Build history of the part. All positions in model axes, mm. Face numbers are marked on the shaded views. A direction names the side the tool comes from. Round coordinates to 2 decimals unless told otherwise and drop trailing zeros. Loops run counter-clockwise (first coordinate to the right, second up) from the corner with the lowest first, then second, coordinate; pieces in that order, holes last. Notation, with made-up numbers: (-35, 4.5) - (13, 4.5) arc R7 ccw to (13, 9.5) - close; hole circle Ø6 at (59, -21.75). An arc over 180 degrees is marked (long way). Put each result on its own line as item: value. Start each with the question number.
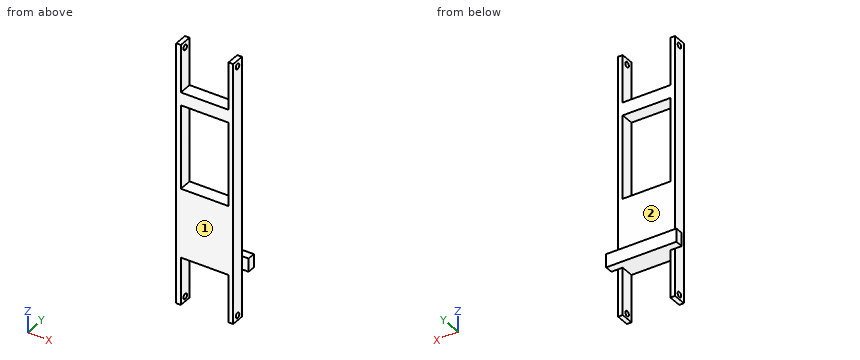
Autodesk Inventor part; units mm, degrees
ref_plane "YZ Plane" through (0, 0, 0) normal (1, 0, 0) x (0, 1, 0)
ref_plane "XZ Plane" through (0, 0, 0) normal (0, 1, 0) x (-1, 0, 0)
ref_plane "XY Plane" through (0, 0, 0) normal (0, 0, 1) x (1, 0, 0)
sketch "Sketch1" plane through (0, 0, 0) normal (0, 1, 0) x (-1, 0, 0)
  line L0 (146.7721, -144.7877) -> (142.3271, -144.7877)
  line L1 (142.3271, -144.7877) -> (142.3271, 134.6123)
  line L2 (142.3271, 134.6123) -> (146.7721, 134.6123)
  line L3 (146.7721, 134.6123) -> (146.7721, -144.7877)
  line L4 (96.6071, -144.7877) -> (96.6071, 134.6123)
  line L5 (96.6071, 134.6123) -> (92.1621, 134.6123)
  line L6 (92.1621, 134.6123) -> (92.1621, -144.7877)
  line L7 (92.1621, -144.7877) -> (96.6071, -144.7877)
  line L8 (142.3271, -91.4477) -> (96.6071, -91.4477)
  line L9 (142.3271, -25.4077) -> (96.6071, -25.4077)
  point P0 (0, 0)
  dimension "d0" = 4.445
  dimension "d1" = 279.4
  dimension "d2" = 4.445
  dimension "d3" = 45.72
  dimension "d4" = 66.04
  dimension "d5" = 53.34
extrude "Extrusion1" add sketch "Sketch1" along normal blind 12.7
sketch "Sketch2" plane through (0, 12.7, 0) normal (0, 1, 0) x (1, 0, 0)
  line L0 (-142.3271, 91.4477) -> (-142.3271, 144.7877)
  line L1 (-142.3271, 91.4477) -> (-146.7721, 91.4477)
  line L2 (-146.7721, 144.7877) -> (-146.7721, -134.6123)
  line L3 (-153.1221, 91.4477) -> (-146.7721, 91.4477)
  line L4 (-96.6071, 91.4477) -> (-142.3271, 91.4477)
  line L5 (-96.6071, 91.4477) -> (-92.1621, 91.4477)
  line L6 (-92.1621, -134.6123) -> (-92.1621, 144.7877)
  line L7 (-92.1621, 91.4477) -> (-85.8121, 91.4477)
  line L8 (-85.8121, 91.4477) -> (-85.8121, 78.7477)
  line L9 (-85.8121, 78.7477) -> (-153.1221, 78.7477)
  line L10 (-153.1221, 78.7477) -> (-153.1221, 91.4477)
  point P0 (0, 0)
  dimension "d8" = 6.35
  dimension "d9" = 6.35
  dimension "d10" = 12.7
extrude "Extrusion2" add sketch "Sketch2" along normal blind 7.62
sketch "Sketch3" plane through (-146.7721, 0, -144.7877) normal (-1, 0, 0) x (0, 0, 1)
  line L0 (279.4, 0) -> (279.4, 12.7)
  circle A0 centre (251.46, 6.35) radius 2.54
  point P0 (144.7877, 0)
  dimension "d15" = 5.08
extrude "Extrusion3" cut sketch "Sketch3" against normal blind 25400
sketch "Sketch4" plane through (-146.7721, 0, -144.7877) normal (-1, 0, 0) x (0, 0, 1)
  line L0 (0, 0) -> (0, 12.7)
  circle A0 centre (12.7052, 6.35) radius 2.54
  point P0 (144.7877, 0)
  dimension "d19" = 5.08
extrude "Extrusion4" cut sketch "Sketch4" against normal blind 25400
sketch "Sketch5" plane through (0, 12.7, 0) normal (0, 1, 0) x (1, 0, 0)
  line L0 (-146.7721, 144.7877) -> (-146.7721, -134.6123)
  line L1 (-142.3271, -134.6123) -> (-142.3271, 25.4077)
  line L2 (-142.3271, -66.9401) -> (-96.6071, -66.9401)
  line L3 (-96.6071, 25.4077) -> (-96.6071, -134.6123)
  line L4 (-96.6071, -54.6023) -> (-142.3271, -54.6023)
  line L5 (-142.3271, -54.6023) -> (-142.3271, -66.9401)
  point P0 (0, 0)
extrude "Extrusion5" add sketch "Sketch5" against normal blind 12.7
sketch "Sketch6" plane through (-146.7721, 0, 134.6123) normal (0, 0, 1) x (1, 0, 0)
  line L0 (0, 12.7) -> (4.445, 12.7)
  line L1 (4.445, 0) -> (4.445, 12.7)
  line L2 (0, 12.7) -> (4.445, 12.7)
  line L3 (4.445, 12.7) -> (4.445, 0)
  line L4 (4.445, 0) -> (0, 0)
  line L5 (0, 0) -> (0, 12.7)
  line L6 (50.165, 0) -> (50.165, 12.7)
  line L7 (54.61, 0) -> (54.61, 12.7)
  line L8 (50.165, 12.7) -> (54.61, 12.7)
  line L9 (54.61, 12.7) -> (54.61, 0)
  line L10 (54.61, 0) -> (50.165, 0)
  line L11 (50.165, 0) -> (50.165, 12.7)
  point P0 (146.7721, 0)
extrude "Extrusion6" cut sketch "Sketch6" against normal blind 22.225
sketch "Sketch7" plane through (-92.1621, 0, -144.7877) normal (0, 0, -1) x (-1, 0, 0)
  line L0 (50.165, 0) -> (50.165, 12.7)
  line L1 (54.61, 12.7) -> (50.165, 12.7)
  line L2 (50.165, 12.7) -> (50.165, 0)
  line L3 (50.165, 0) -> (54.61, 0)
  line L4 (54.61, 0) -> (54.61, 12.7)
  line L5 (4.445, 0) -> (4.445, 12.7)
  line L6 (0, 0) -> (4.445, 0)
  line L7 (4.445, 12.7) -> (0, 12.7)
  line L8 (0, 12.7) -> (0, 0)
  line L9 (0, 0) -> (4.445, 0)
  line L10 (4.445, 0) -> (4.445, 12.7)
  point P0 (-92.1621, 0)
extrude "Extrusion7" cut sketch "Sketch7" against normal blind 7.9375
properties part number "Mousetrap Car"
1) Slice it at C-C, the plane z = 7. Write the cut outline in (x, y).
2) Slice it at D-D, the plane y = 17.25. Write the cut outline in (x, z).
3) Slice it at B-B, the plane x = -101.5. Write the cut outline in (y, z), and give its area (3 significant figures).
4) Slice it at A-A, the plane y = 6.35. State how many separate pieces and enclosed holes the cut face has, and give its area (3 significant figures).
5) Drill centre lines: line 1 (Z direction, x = -100.5, y = 3.5); line 2 (X direction, y = 7, z = 89); line 3 (Y direction, x = -102.5, z = -66). Where is each one in solid material? Low to high. Write a range as [from, to].
6) Drop flat-ended pins along their axis: pin 1 Ø6.5 at (y, z) = (6, 25) entering from +X; pin 2 Ø10 at (x, y) = (-126.5, 5) entering from -Z; pin 3 Ø2 at (x, y) = (-124.5, 17.5) entering from +Z; pin 4 Ø4 at (y, z) = (6.35, -132.08) entering from +X. Give the stop position or say it passes through.
7) Which spindle directions (+Z, -Z, +X, -X, +Y, -Y) get a long thin tool onto all of the face, cutting with end or side? Do the marked faces 1 and 2. Say none if no direction does.
Taken from the geometry:
1. outline: (-146.77, 0) - (-142.33, 0) - (-142.33, 12.7) - (-146.77, 12.7) - close; (-96.61, 0) - (-92.16, 0) - (-92.16, 12.7) - (-96.61, 12.7) - close
2. outline: (-153.12, -91.45) - (-85.81, -91.45) - (-85.81, -78.75) - (-153.12, -78.75) - close
3. outline: (0, -91.45) - (20.32, -91.45) - (20.32, -78.75) - (12.7, -78.75) - (12.7, -25.41) - (0, -25.41) - close; (0, 54.6) - (12.7, 54.6) - (12.7, 66.94) - (0, 66.94) - close
3. area: 1,090 mm2
4. separate pieces: 5
4. enclosed holes: 1
4. area: 5,710 mm2
5. line 1: z = [-91.45, -25.41], [54.6, 66.94]
5. line 2: x = [-146.77, -142.33], [-96.61, -92.16]
5. line 3: y = [0, 12.7]
6. pin 1: stops at x = -92.16
6. pin 2: stops at z = -91.45
6. pin 3: stops at z = -78.75
6. pin 4: passes through
7. face 1: +Z, -Z, +X, -X, -Y
7. face 2: +Z, +X, -X, +Y
